from build123d import *

# Parameters (mm, degrees)
SKETCH1_W           = 70
SKETCH1_H           = 70
BOSS_EXTRUDE1_DEPTH = 25
SKETCH2_R           = 2.2
CUT_EXTRUDE1_DEPTH  = 56.452682532
FILLET1_R           = 4


with BuildPart() as part:
    # Sketch1 → Boss-Extrude1 (new body)
    with BuildSketch(Plane.XY):
        Rectangle(SKETCH1_W, SKETCH1_H)
    extrude(amount=BOSS_EXTRUDE1_DEPTH)

    # Sketch2 → Cut-Extrude1 (cut, through all)
    with BuildSketch(Plane.XY.offset(25)):
        with Locations((-30.8, 30.8)):
            Circle(SKETCH2_R)
        with Locations((30.8, 30.8)):
            Circle(SKETCH2_R)
        with Locations((30.8, -30.8)):
            Circle(SKETCH2_R)
        with Locations((-30.8, -30.8)):
            Circle(SKETCH2_R)
    extrude(amount=-CUT_EXTRUDE1_DEPTH, mode=Mode.SUBTRACT)

    # Fillet1
    fillet1_edges = [part.edges().sort_by_distance(p)[0] for p in [
        (35, -35, 12.5),
        (-35, -35, 12.5),
        (-35, 35, 12.5),
        (35, 35, 12.5),
    ]]
    fillet(fillet1_edges, radius=FILLET1_R)


solid = part.part
Could you check a few things on this model? Use its own coordinates, in mm. Coordinates: 2 decimals unless noted, no trailing zeros. Order: outer loops, then holes, each group sorted by start corner. A loop starts at its lowest first (then second) coordinate and runs counter-clockwise, first axis right, second up.
Q1. Please list where this line runs through material, in increasing order: L1, parallel to Y at x = 30.8, z = 10.
Q2. Suppose I cut it at A-A on z = 23.25. Please give me the cut outline in (x, y), and give its area (3 significant figures).
Q3. Thinking about a two-plate mould opening in Y: for faces 1 (the flat face through (0, -35, 12)), 2 (the flat face through (0, 35, 12)), 3 (the cylindrical face through (-32.998, 30.897, 12.675)), 4 (the flat face through (35, 0, 12)), which applies, released by +Y, released by -Y, zero draft, split by the parting line, or undercut?
Answer:
1. L1: y = -35 to -33, -28.6 to 28.6, 33 to 35
2. outline: (-35, -31) arc R4 ccw to (-31, -35) - (31, -35) arc R4 ccw to (35, -31) - (35, 31) arc R4 ccw to (31, 35) - (-31, 35) arc R4 ccw to (-35, 31) - close; hole circle Ø4.4 at (-30.8, -30.8); hole circle Ø4.4 at (-30.8, 30.8); hole circle Ø4.4 at (30.8, -30.8); hole circle Ø4.4 at (30.8, 30.8)
2. area: 4,830 mm2
3. face 1: released by -Y
3. face 2: released by +Y
3. face 3: undercut
3. face 4: zero draft
